Here's how the part is built. I have some questions about the finished solid (model axes, mm). Round coordinates to 2 decimals unless told otherwise and drop trailing zeros. Write each loop counter-clockwise with the first axis right and the second up, starting at its lowest first coordinate (ties: lowest second). Pieces come first, ordered by that corner, then holes. Notation, with made-up numbers: (-35, 13.25) -> (-18, 13.25) arc R19 cw to (-18, 46.25) -> close; hole circle Ø1 at (-25.75, -31). An arc over 180 degrees is marked (long way). Answer in a Markdown table with one row per item.
from build123d import *

# Parameters (mm, degrees)
SKETCH1_R           = 75
BOSS_EXTRUDE1_DEPTH = 10
CUT_EXTRUDE1_DEPTH  = 10
LPATTERN1_DEPTH     = 10
CIRPATTERN1_COUNT   = 4


# Read off the part's stored shape, not the designer's step: LPattern1
with BuildPart() as part:
    # Sketch1 → Boss-Extrude1 (new body)
    with BuildSketch(Plane.XY):
        Circle(SKETCH1_R)
    extrude(amount=BOSS_EXTRUDE1_DEPTH)

    # Sketch2 → Cut-Extrude1 (cut)
    with BuildSketch(Plane.XY.offset(10)):
        with BuildLine():
            ThreePointArc((35, 60.621778265), (0, 70), (-35, 60.621778265))
            ThreePointArc((-35, 60.621778265), (-36.830127019, 53.791651246), (-30, 51.961524227))
            ThreePointArc((-30, 51.961524227), (0, 60), (30, 51.961524227))
            ThreePointArc((30, 51.961524227), (36.830127019, 53.791651246), (35, 60.621778265))
        make_face()
    cut_extrude1 = extrude(amount=-CUT_EXTRUDE1_DEPTH, mode=Mode.SUBTRACT)

    # LPattern1 outline → LPattern1 (cut)
    with BuildSketch(Plane.XY):
        with BuildLine():
            ThreePointArc((-22.5, 38.97114317), (0, 45), (22.5, 38.97114317))
            ThreePointArc((22.5, 38.97114317), (29.330127019, 40.801270189), (27.5, 47.631397208))
            ThreePointArc((27.5, 47.631397208), (0, 55), (-27.5, 47.631397208))
            ThreePointArc((-27.5, 47.631397208), (-29.330127019, 40.801270189), (-22.5, 38.97114317))
        make_face()
        with BuildLine():
            ThreePointArc((-7.5, 12.990381057), (0, 15), (7.5, 12.990381057))
            ThreePointArc((7.5, 12.990381057), (14.330127019, 14.820508076), (12.5, 21.650635095))
            ThreePointArc((12.5, 21.650635095), (0, 25), (-12.5, 21.650635095))
            ThreePointArc((-12.5, 21.650635095), (-14.330127019, 14.820508076), (-7.5, 12.990381057))
        make_face()
        with BuildLine():
            ThreePointArc((-15, 25.980762114), (0, 30), (15, 25.980762114))
            ThreePointArc((15, 25.980762114), (21.830127019, 27.810889132), (20, 34.641016151))
            ThreePointArc((20, 34.641016151), (0, 40), (-20, 34.641016151))
            ThreePointArc((-20, 34.641016151), (-21.830127019, 27.810889132), (-15, 25.980762114))
        make_face()
    lpattern1 = extrude(amount=LPATTERN1_DEPTH, mode=Mode.SUBTRACT)

    # CirPattern1: Cut-Extrude1, LPattern1 ×4 about axis
    cirpattern1_axis = Axis((0, 0, 0), (0, 0, 1))
    add([cut_extrude1.rotate(cirpattern1_axis, i * 360 / CIRPATTERN1_COUNT) for i in range(1, CIRPATTERN1_COUNT)], mode=Mode.SUBTRACT)
    add([lpattern1.rotate(cirpattern1_axis, i * 360 / CIRPATTERN1_COUNT) for i in range(1, CIRPATTERN1_COUNT)], mode=Mode.SUBTRACT)


solid = part.part
1) For pin 1 (2 mm diameter, centred on y = 30, z = 6.5, fed in from -X); pin 2 (5 mm diameter, centred on x = -9.5, z = 7.5, fed in from -Y); pin 3 (6 mm diameter, centred on x = 17.5, z = 3.5, fed in from -Y) (3 decimals), each with a flat end and sliding along its axis, tell me the tip position at first contact or that it passes through.
Response:
| item | result |
|---|---|
| pin 1 | stops at x = -69.17 |
| pin 2 | stops at y = -74.67 |
| pin 3 | stops at y = -73.585 |
2) I want a section at C-C, the plane y = -32.5. List the corners of the cut face in (x, z) for me.
Response:
| item | result |
|---|---|
| outline | (-67.59, 0) -> (-62, 0) -> (-62, 10) -> (-67.59, 10) -> close; (-51.29, 0) -> (-22, 0) -> (-22, 10) -> (-51.29, 10) -> close; (22, 0) -> (51.29, 0) -> (51.29, 10) -> (22, 10) -> close; (62, 0) -> (67.59, 0) -> (67.59, 10) -> (62, 10) -> close |
3) We'd pull the mould along Y, two halves only. Please class faces 1 (the face through (-9.764, 74.362, 4.93)), 2 (the face through (55, 0, 5)): +Y half, -Y half, draft (parallel to the pull), parting line (faces both ways), or undercut.
Response:
| item | result |
|---|---|
| face 1 | parting line |
| face 2 | undercut |
4) I want a section at A-A, the plane x = 17.5. Count the separate pieces of the cut face and the enclosed holes in it, and give its area (3 significant figures).
Response:
| item | result |
|---|---|
| separate pieces | 8 |
| enclosed holes | 0 |
| area | 524 mm^2 |
5) I need wall thicknesses on line 1 (X direction, y = -33, z = 1); line 2 (X direction, y = 45.5, z = 3). Which ranges of each line are inside material? Lowest first, please. Write a range as [from, to].
Response:
| item | result |
|---|---|
| line 1 | x = [-67.35, -61.73], [-51.32, -21.72], [21.72, 51.32], [61.73, 67.35] |
| line 2 | x = [-59.62, -29.49], [29.49, 59.62] |
